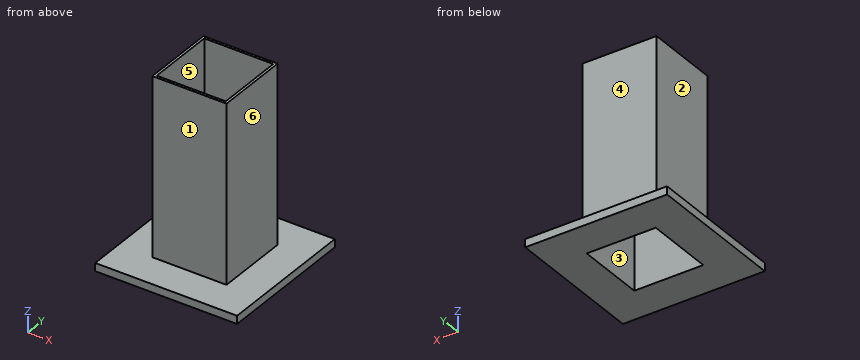
```python
from build123d import *

# Parameters (mm, degrees)
SKETCH_W     = 88
SKETCH_H     = 88
PAD_DEPTH    = 5
SKETCH001_W  = 46
SKETCH001_H  = 46
PAD001_DEPTH = 110
SKETCH002_W  = 42.8
SKETCH002_H  = 42.8
POCKET_DEPTH = 115.001


with BuildPart() as part:
    # Sketch → Pad (new body)
    with BuildSketch(Plane.XY):
        Rectangle(SKETCH_W, SKETCH_H)
    extrude(amount=PAD_DEPTH)

    # Sketch001 (on Face6 of Pad) → Pad001 (join)
    with BuildSketch(Plane.XY.offset(5)):
        Rectangle(SKETCH001_W, SKETCH001_H)
    extrude(amount=PAD001_DEPTH)

    # Sketch002 (on Face11 of Pad001) → Pocket (cut, through all)
    with BuildSketch(Plane.XY.offset(115)):
        Rectangle(SKETCH002_W, SKETCH002_H)
    extrude(amount=-POCKET_DEPTH, mode=Mode.SUBTRACT)


solid = part.part
```
Verification items for the finished model (mm, model axes). Face numbers are marked on the shaded views. A direction names the side the tool comes from. Round coordinates to 2 decimals unless told otherwise and drop trailing zeros. Write each loop counter-clockwise with the first axis right and the second up, starting at its lowest first coordinate (ties: lowest second). Pieces come first, ordered by that corner, then holes.
1. Section check B-B on z = 17. Enter the section's corners in (x, y).
2. Access from +Z, -Z, +X, -X, +Y, -Y to the whole of each face (thin tool, end or side, straight path). Record for the marked faces 4, 5 and 6.
3. Scan lines: L1, parallel to Y at x = 9, z = 30; L2, parallel to Z at x = -38, y = -11.5. Record each from-to range of solid material in increasing order.
4. Draft check along Y on the marked faces 1, 2 and 3. Enter one of: +Y half, -Y half, draft (parallel to the pull), parting line (faces both ways), or undercut.
5. Section check A-A on x = 5. Enter the section's corners in (y, z).
6. Section check D-D on x = 28.5. Enter the section's corners in (y, z), plus the area to 3 significant figures.
7. Gauge pin test, flat ends, axial feed: P1, Ø12, axis at x = 17, y = 21.5, coming from the -Z side; P2, Ø23, axis at x = 0.5, z = 49, coming from the +Y side; P3, Ø14, axis at y = -3.5, z = 54, coming from the -X side; P4, Ø12, axis at x = 24, y = 29.5, coming from the +Z side. Record the tip position at first contact, or that the pin passes through.
Answer:
1. outline: (-23, -23) - (23, -23) - (23, 23) - (-23, 23) - close; hole (-21.4, -21.4) - (21.4, -21.4) - (21.4, 21.4) - (-21.4, 21.4) - close
2. face 4: +Z, +X, -X, +Y
2. face 5: +Z, -Z
2. face 6: +Z, +X, +Y, -Y
3. L1: y = -23 to -21.4, 21.4 to 23
3. L2: z = 0 to 5
4. face 1: -Y half
4. face 2: draft
4. face 3: undercut
5. outline: (-44, 0) - (-21.4, 0) - (-21.4, 115) - (-23, 115) - (-23, 5) - (-44, 5) - close; (21.4, 0) - (44, 0) - (44, 5) - (23, 5) - (23, 115) - (21.4, 115) - close
6. outline: (-44, 0) - (44, 0) - (44, 5) - (-44, 5) - close
6. area: 440 mm2
7. P1: stops at z = 0
7. P2: stops at y = 23
7. P3: stops at x = -23
7. P4: stops at z = 5
